Work out the finished part from the listing and answer in its coordinate system (mm). A direction names the side the tool comes from. Round coordinates to 2 decimals unless told otherwise and drop trailing zeros. Loops run counter-clockwise (first coordinate to the right, second up) from the corner with the lowest first, then second, coordinate; pieces in that order, holes last. Notation, with made-up numbers: M 16.25,0.5 L 45.25,0.5 A14 cw 45.25,25.5 Z; hole C 45.5,55 d5. An arc over 180 degrees is marked long. One line per item, written item: value.
```python
from build123d import *

# Parameters (mm, degrees)
BOSS_EXTRU_1_DEPTH      = 7
D_GAGEMENT_M31_DEPTH    = 7
BOSS_EXTRU_3_DEPTH      = 7
BOSS_EXTRU_4_DEPTH      = 16
ESQUISSE8_R             = 15
ENL_V_MAT_EXTRU_1_DEPTH = 4
ESQUISSE9_R             = 6.5
BOSS_EXTRU_5_DEPTH      = 0.5
D_GAGEMENT_M51_D        = 5.5
ESQUISSE12_R            = 6.5
BOSS_EXTRU_6_DEPTH      = 3.7


# Read off the part's stored shape, not the designer's step: Dégagement M31
with BuildPart() as part:
    # Esquisse1 → Boss.-Extru.1 (new body)
    with BuildSketch(Plane(origin=(0, 0, 0), x_dir=(0, 0, -1), z_dir=(1, 0, 0))):
        with BuildLine():
            Line((8, 4), (8, -4))
            ThreePointArc((8, -4), (0, -12), (-8, -4))
            Line((-8, -4), (-8, 4))
            ThreePointArc((-8, 4), (0, 12), (8, 4))
        make_face()
    extrude(amount=BOSS_EXTRU_1_DEPTH)

    # Dégagement M31 outline → Dégagement M31 (cut)
    with BuildSketch(Plane.YZ):
        with BuildLine():
            Line((-2.45, -1.7), (2.45, -1.7))
            ThreePointArc((2.45, -1.7), (4.15, 0), (2.45, 1.7))
            Line((2.45, 1.7), (-2.45, 1.7))
            ThreePointArc((-2.45, 1.7), (-4.15, 0), (-2.45, -1.7))
        make_face()
    extrude(amount=D_GAGEMENT_M31_DEPTH, mode=Mode.SUBTRACT)

    # Esquisse6 → Boss.-Extru.3 (add, through all)
    with BuildSketch(Plane(origin=(7, 0, 0), x_dir=(0, 0, -1), z_dir=(1, 0, 0))):
        with BuildLine():
            ThreePointArc((-5e-09, -12), (-5.656854251, -9.656854248), (-8, -4))
            Line((-8, -4), (-8, -12))
            Line((-8, -12), (-5e-09, -12))
        make_face()
        with BuildLine():
            ThreePointArc((8, -4), (5.656854248, -9.656854251), (-5e-09, -12))
            Line((-5e-09, -12), (8, -12))
            Line((8, -12), (8, -4))
        make_face()
    extrude(amount=-BOSS_EXTRU_3_DEPTH)

    # Esquisse7 → Boss.-Extru.4 (add, through all)
    with BuildSketch(Plane.XY.offset(8)):
        with BuildLine():
            Line((3.307940197, -29.244206061), (0, -12))
            Line((0, -12), (7, -12))
            Line((7, -12), (7, -7.5))
            Line((7, -7.5), (15.544704758, -25.192887251))
            ThreePointArc((15.544704758, -25.192887251), (11.734497019, -34.190248899), (3.307940197, -29.244206061))
        make_face()
    extrude(amount=-BOSS_EXTRU_4_DEPTH)

    # Esquisse8 → Enlèv. mat.-Extru.1 (cut, symmetric)
    with BuildSketch(Plane.XY):
        with Locations((9.69154802, -28.01964444)):
            Circle(ESQUISSE8_R)
    extrude(amount=ENL_V_MAT_EXTRU_1_DEPTH, both=True, mode=Mode.SUBTRACT)

    # Esquisse9 → Boss.-Extru.5 (add)
    with BuildSketch(Plane(origin=(0, 0, 4), x_dir=(-1, 0, 0), z_dir=(0, 0, -1))):
        with Locations(Location((-9.69154802, -28.01964444, 0), (0, 0, 154.221977628))):
            Circle(ESQUISSE9_R)
    boss_extru_5 = extrude(amount=BOSS_EXTRU_5_DEPTH)

    # Symétrie1: Boss.-Extru.5 across plane
    add(boss_extru_5.mirror(Plane.XY))

    # Dégagement M51 (through all)
    with Locations(Plane.XY.offset(8)):
        with Locations((9.69154802, -28.01964444)):
            Hole(D_GAGEMENT_M51_D / 2)

    # Esquisse12 → Boss.-Extru.6 (add)
    with BuildSketch(Plane(origin=(0, 0, -8), x_dir=(-1, 0, 0), z_dir=(0, 0, -1))):
        with Locations(Location((-9.69154802, -28.01964444, 0), (0, 0, 90))):
            Circle(ESQUISSE12_R)
        Polygon((-4.668600678, -28.01964444), (-7.180074349, -23.66964444), (-12.203021691, -23.66964444), (-14.714495362, -28.01964444), (-12.203021691, -32.36964444), (-7.180074349, -32.36964444), align=None, mode=Mode.SUBTRACT)
    extrude(amount=BOSS_EXTRU_6_DEPTH)


solid = part.part
```
1) Find section A-A (y = 1.5). Give the vertices of the cut face in (x, z), then the cut area to 3 significant figures.
Check values:
outline: M 0,-8 L 7,-8 L 7,-1.7 L 0,-1.7 Z; M 0,1.7 L 7,1.7 L 7,8 L 0,8 Z
area: 88.2 mm2
2) For faces 1 (the face through (12, -26, 3.5)), 2 (the face through (7, 2, 2)), 3 (the face through (13.44, -25.81, -9.82)), determine the directions among +Z, -Z, +X, -X, +Y, -Y from which every point of the face is accessible in a straight line to the end or side of a thin tool.
Check values:
face 1: +X, -X, -Y
face 2: +Z, -Z, +X, +Y
face 3: -Z
3) Find the intervals of material crossed by probe 1 along Z at (x, y) = (7.25, -16.5); probe 2 along X at (y, z) = (-2.5, 3.25); probe 3 along Y at (x, z) = (11.75, -8.5), in increasing order. Write a range as from..to.
Check values:
probe 1: -8..-4, 4..8
probe 2: 0..7
probe 3: -34.19..-32.37, -23.67..-21.85
4) Find section D-D (x = 13.25). Give the vertices of the cut face in (y, z).
Check values:
outline: M -33.46,-11.7 L -30.56,-11.7 L -30.56,-8 L -25.48,-8 L -25.48,-11.7 L -22.58,-11.7 L -22.58,-8 L -20.44,-8 L -20.44,-4 L -22.58,-4 L -22.58,-3.5 L -33.46,-3.5 Z; M -33.46,3.5 L -22.58,3.5 L -22.58,4 L -20.44,4 L -20.44,8 L -33.46,8 Z
5) Find section C-C (z = -7.5). Give the vertices of the cut face in (x, y).
Check values:
outline: M 0,-12 L 3.31,-29.24 A6.5 ccw long 15.54,-25.19 L 7,-7.5 L 7,6.78 L 0,6.78 Z; hole C 9.69,-28.02 d5.5
6) The mould has two halves that part along Z. Classify faces 4 (the face through (7.07, -27.19, 5.72)), 5 (the face through (6, -19, 4)), 6 (the face through (7.5, -26, -8)): +Z half, -Z half, draft (parallel to the pull), parting line (faces both ways), or undercut.
Check values:
face 4: draft
face 5: undercut
face 6: -Z half
7) Find section B-B (z = 0). Give the vertices of the cut face in (x, y).
Check values:
outline: M 0,-12 L 0.76,-15.97 A15 cw 9.67,-13.02 L 7,-7.5 L 7,-4.15 L 0,-4.15 Z; M 0,4.15 L 7,4.15 L 7,12 L 0,12 Z
8) Each of these flat-tipped pins is pushed along its axis until it touches: pin 1 (1.5 mm diameter, centred on x = 4.5, y = 0.5, fed in from -Z); pin 2 (2 mm diameter, centred on y = 0, z = -1.5, fed in from +X); pin 3 (1.8 mm diameter, centred on x = 9.5, z = -9, fed in from +Y). Where does it stop, or does it pass through?
Check values:
pin 1: z = -8
pin 2: x = 7
pin 3: y = -21.52
